Design review of the part shown in the three views and the two pictorial views. Dimensions are in mm from the part's minimum x, y and z. A direction names the side the tool comes from. Coordinates: 2 decimals unless noted, no trailing zeros. Loops run counter-clockwise (first coordinate to the right, second up) from the corner with the lowest first, then second, coordinate; pieces in that order, holes last. Notation, with made-up numbers: (-23, 35.5) -> (8, 35.5) arc R4 ccw to (8, 41.5) -> close; hole circle Ø6 at (-39, -32.75). An arc over 180 degrees is marked (long way). One line per item, written item: value. Start each with the question number.
1. Add section B-B on y = 3. Write out the cut boundary in (x, z).
2. Machinability: for the marked faces 1, 2 and 3, which of the approach directions +Z, -Z, +X, -X, +Y, -Y give a long, thin tool a straight path to every point of the face, cutting with its end or side? Answer none if there is none.
3. Add section C-C on z = 38.85. Write out the cut boundary in (x, y).
4. Insertion check: pin 1 (6 mm diameter, centred on x = 4.5, y = 5, fed in from -Z); pin 2 (1.5 mm diameter, centred on y = 6, z = 9.5, fed in from +X); pin 3 (2 mm diameter, centred on y = 4.5, z = 30, fed in from +X). Each pin has a flat end and moves straight along its axis. Give the tip position at first contact, or say it passes through.
5. Draft analysis for pull direction Z (two halves, no side actions). For the marked faces 4, 5 and 6, state which applies: pulls with the +Z half, pulls with the -Z half, needs draft (parallel to the pull), parting line crosses it, or undercut.
6. For probe 1 along X at (y, z) = (0.8, 6.6); probe 2 along Z at (x, y) = (13, 7); probe 3 along Z at (x, y) = (18.6, 0.45), list the stretches that pass through material, from the lowest coordinate up.
7. Add section D-D on y = 9.75. Write out the cut boundary in (x, z), plus the area to 3 significant figures.
8. Add section A-A on x = 2.6. Write out the cut boundary in (y, z), plus the area to 3 significant figures.
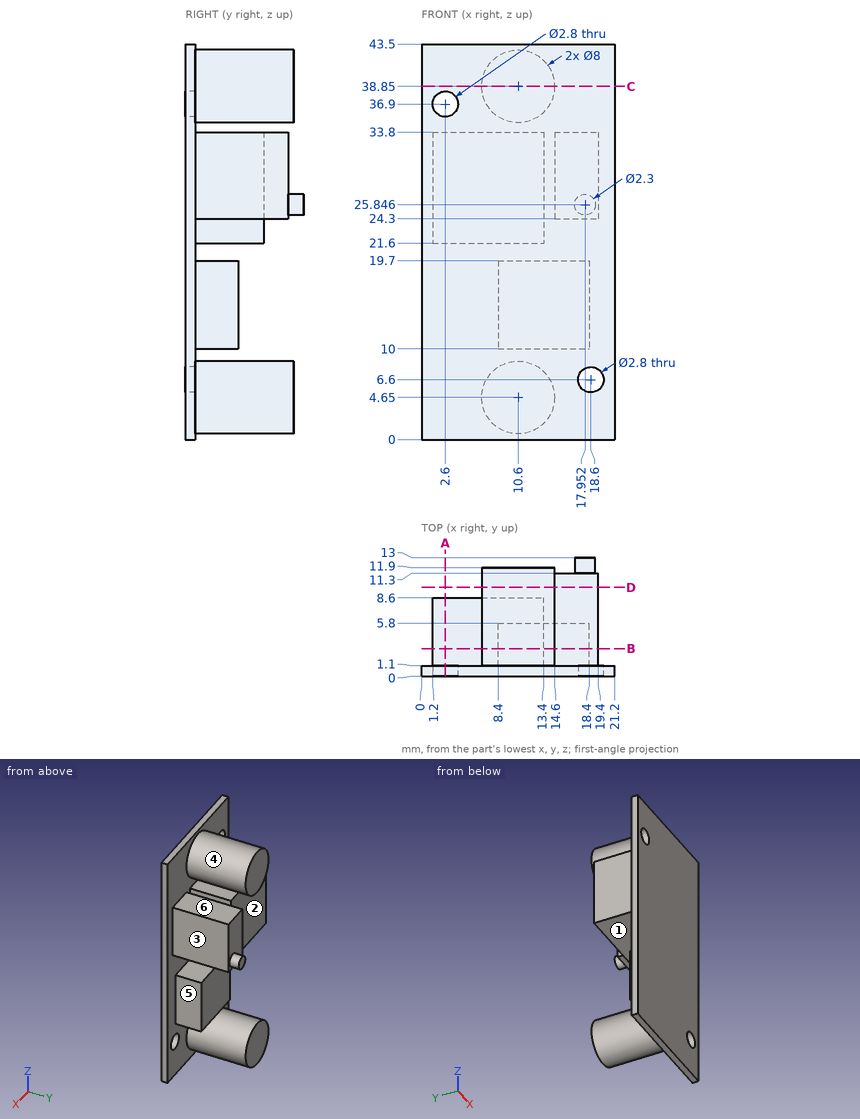
Worked answers:
1. outline: (1.2, 21.6) -> (13.4, 21.6) -> (13.4, 33.8) -> (1.2, 33.8) -> close; circle Ø8 at (10.6, 4.65); circle Ø8 at (10.6, 38.85); (8.4, 10) -> (18.4, 10) -> (18.4, 19.7) -> (8.4, 19.7) -> close; (14.6, 24.3) -> (19.4, 24.3) -> (19.4, 33.8) -> (14.6, 33.8) -> close
2. face 1: +X, -X, +Y
2. face 2: -X, +Y
2. face 3: +Z, -Z, +X, +Y
3. outline: (0, 0) -> (21.2, 0) -> (21.2, 1.1) -> (14.6, 1.1) -> (14.6, 11.9) -> (6.6, 11.9) -> (6.6, 1.1) -> (0, 1.1) -> close
4. pin 1: stops at z = 2.12
4. pin 2: stops at x = 18.4
4. pin 3: stops at x = 19.4
5. face 4: undercut
5. face 5: needs draft
5. face 6: pulls with the +Z half
6. probe 1: x = 0 to 17.2, 20 to 21.2
6. probe 2: z = 1.45 to 7.85, 21.6 to 33.8, 35.65 to 42.05
6. probe 3: z = 0 to 5.2, 8 to 43.5
7. outline: circle Ø8 at (10.6, 4.65); circle Ø8 at (10.6, 38.85); (14.6, 24.3) -> (19.4, 24.3) -> (19.4, 33.8) -> (14.6, 33.8) -> close
7. area: 146 mm²
8. outline: (0, 0) -> (1.1, 0) -> (1.1, 21.6) -> (8.6, 21.6) -> (8.6, 33.8) -> (1.1, 33.8) -> (1.1, 35.5) -> (0, 35.5) -> close; (0, 38.3) -> (1.1, 38.3) -> (1.1, 43.5) -> (0, 43.5) -> close
8. area: 136 mm²
